from build123d import *

# Parameters (mm, degrees)
SKETCH1_R           = 32
BOSS_EXTRUDE1_DEPTH = 4
SKETCH2_R           = 5
CUT_EXTRUDE1_DEPTH  = 5
CIRPATTERN1_COUNT   = 6
BOSS_EXTRUDE2_DEPTH = 32
CHAMFER1_SIZE       = 2
CHAMFER2_SIZE       = 0.2
SKETCH4_R           = 6
CUT_EXTRUDE2_DEPTH  = 32
CHAMFER3_SIZE       = 0.6
CHAMFER4_SIZE       = 5
CHAMFER5_SIZE       = 2


with BuildPart() as part:
    # Sketch1 → Boss-Extrude1 (new body)
    with BuildSketch(Plane.XY):
        Circle(SKETCH1_R)
    extrude(amount=-BOSS_EXTRUDE1_DEPTH)

    # Sketch2 → Cut-Extrude1 (cut, through all)
    with BuildSketch(Plane.XY):
        with Locations((0, 24)):
            Circle(SKETCH2_R)
    cut_extrude1 = extrude(amount=-CUT_EXTRUDE1_DEPTH, mode=Mode.SUBTRACT)

    # CirPattern1: Cut-Extrude1 ×6 about axis
    cirpattern1_axis = Axis((0, 0, 0), (0, 0, 1))
    for i in range(1, CIRPATTERN1_COUNT):
        add(cut_extrude1.rotate(cirpattern1_axis, i * 360 / CIRPATTERN1_COUNT), mode=Mode.SUBTRACT)

    # Sketch3 → Boss-Extrude2 (add)
    with BuildSketch(Plane(origin=(0, 0, -4), x_dir=(-1, 0, 0), z_dir=(0, 0, -1))):
        Polygon((-4.618802154, 8), (-9.237604307, 0), (-4.618802154, -8), (4.618802154, -8), (9.237604307, 0), (4.618802154, 8), align=None)
    extrude(amount=BOSS_EXTRUDE2_DEPTH)

    # Chamfer1
    chamfer1_edges = [part.edges().sort_by_distance(p)[0] for p in [
        (0, 8, -4),
        (6.92820323, 4, -4),
        (6.92820323, -4, -4),
        (0, -8, -4),
        (-6.92820323, -4, -4),
        (-6.92820323, 4, -4),
    ]]
    chamfer(chamfer1_edges, length=CHAMFER1_SIZE)

    # Chamfer2
    chamfer2_edges = [part.edges().sort_by_distance(p)[0] for p in [
        (-23.284609691, 7.669872981, -4),
        (-18.284609691, -16.330127019, -4),
        (5, -24, -4),
        (23.284609691, -7.669872981, -4),
        (18.284609691, 16.330127019, -4),
        (-32, 0, -4),
        (-5, 24, -4),
    ]]
    chamfer(chamfer2_edges, length=CHAMFER2_SIZE)

    # Sketch4 → Cut-Extrude2 (cut)
    with BuildSketch(Plane.XY):
        Circle(SKETCH4_R)
    extrude(amount=-CUT_EXTRUDE2_DEPTH, mode=Mode.SUBTRACT)

    # Chamfer3
    chamfer3_edges = [part.edges().sort_by_distance(p)[0] for p in [
        (0, 8, -36),
        (6.92820323, 4, -36),
        (6.92820323, -4, -36),
        (0, -8, -36),
        (-6.92820323, -4, -36),
        (-6.92820323, 4, -36),
    ]]
    chamfer(chamfer3_edges, length=CHAMFER3_SIZE)

    # Chamfer4
    chamfer4_edges = [part.edges().sort_by_distance(p)[0] for p in [
        (-6, 0, -32),
    ]]
    chamfer(chamfer4_edges, length=CHAMFER4_SIZE)

    # Chamfer5
    chamfer5_edges = [part.edges().sort_by_distance(p)[0] for p in [
        (-6, 0, 0),
    ]]
    chamfer(chamfer5_edges, length=CHAMFER5_SIZE)


solid = part.part
Design review of the part built by this model. Coordinates are the model's own, in mm. A direction names the side the tool comes from. Give positions to 0.01 mm unless a question says otherwise; leave off trailing zeros. Order: outer loops, then holes, each group sorted by start corner. A loop starts at its lowest first (then second) coordinate and runs counter-clockwise, first axis right, second up. Notation, with made-up numbers: (-4.75, 55.5) - (24.25, 55.5) arc R26 cw to (24.25, 82.5) - close; hole circle Ø9 at (63.5, 63). An arc over 180 degrees is marked (long way). Use CSV: the item, a comma, the result in double quotes. Start each with the question number.
Q1. Take a section at A-A (x = 0). Count the separate pieces of the cut face and the enclosed holes in it, and give its area (3 significant figures).
Q2. Take a section at B-B (z = -15.5). State the section outline as (x, y) points.
Q3. For P1, Ø10, axis at x = 5, z = -27.5, coming from the -Y side; P2, Ø3, axis at x = 10.5, z = -20.5, coming from the -Y side; P3, Ø7.5, axis at x = 1.5, z = -19.5, coming from the +Y side, all flat-tipped, find the tip position at first contact; note any pin that passes through.
Q4. Take a section at C-C (z = -3). State the section outline as (x, y) points, and give its area (3 significant figures).
Q5. Draft analysis for pull direction X (two halves, no side actions). For faces 1 (the face through (16.016, 10.498, -1.873)), 2 (the face through (0, 8, -20)), 3 (the face through (6.632, 3.904, -35.704)), state which applies: pulls with the +X half, pulls with the -X half, needs draft (parallel to the pull), parting line crosses it, or undercut.
Q6. For line 1 (Y direction, x = 0, z = -2.85); line 2 (Y direction, x = 0, z = -16); line 3 (Z direction, x = 10.5, y = -17), list the stretches that pass through material, from the lowest coordinate up.
Q7. Machinability: for faces 4 (the face through (-6.896, -4.056, -20.494)), 5 (the face through (-6.961, 3.944, -20.494)), 6 (the face through (6.961, -3.944, -20.494)), 7 (the face through (-6, 0, -14)), which of the approach directions +Z, -Z, +X, -X, +Y, -Y give a long, thin tool a straight path to every point of the face, cutting with its end or side? Answer none if there is none.
Calculated:
1,separate pieces,"3"
1,enclosed holes,"0"
1,area,"329 mm²"
2,outline,"(-9.24, 0) - (-4.62, -8) - (4.62, -8) - (9.24, 0) - (4.62, 8) - (-4.62, 8) - close; hole circle Ø12 at (0, 0)"
3,P1,"stops at y = -8"
3,P2,"stops at y = -0.41"
3,P3,"stops at y = 8"
4,outline,"circle Ø64 at (0, 0); hole circle Ø10 at (-20.78, -12); hole circle Ø10 at (-20.78, 12); hole circle Ø12 at (0, 0); hole circle Ø10 at (0, -24); hole circle Ø10 at (0, 24); hole circle Ø10 at (20.78, -12); hole circle Ø10 at (20.78, 12)"
4,area,"2,630 mm²"
5,face 1,"undercut"
5,face 2,"needs draft"
5,face 3,"pulls with the +X half"
6,line 1,"y = -32 to -29, -19 to -6, 6 to 19, 29 to 32"
6,line 2,"y = -8 to -6, 6 to 8"
6,line 3,"z = -4 to 0"
7,face 4,"-Z, -X, -Y"
7,face 5,"-Z, -X, +Y"
7,face 6,"-Z, +X, -Y"
7,face 7,"+Z"
